Check sheet for the modelled part. Datum: model origin and axes. Units: mm. Face numbers are marked on the shaded views. Give positions to 0.01 mm unless a question says otherwise; leave off trailing zeros. Write each loop counter-clockwise with the first axis right and the second up, starting at its lowest first coordinate (ties: lowest second). Pieces come first, ordered by that corner, then holes. Notation, with made-up numbers: (-19, 58.25) -> (2, 58.25) arc R27 cw to (2, 84.25) -> close; hole circle Ø3 at (-34.75, 57.25). An arc over 180 degrees is marked (long way). Return JSON: item names as keys, results as strings.
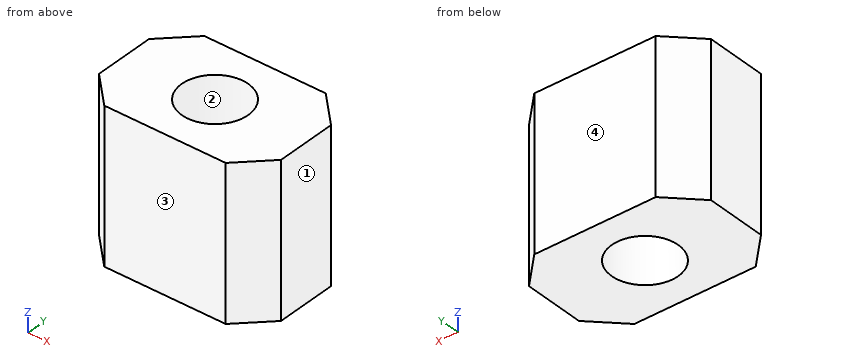
Autodesk Inventor part; units mm, degrees
ref_plane "YZ Plane" through (0, 0, 0) normal (1, 0, 0) x (0, 1, 0)
ref_plane "XZ Plane" through (0, 0, 0) normal (0, 1, 0) x (-1, 0, 0)
ref_plane "XY Plane" through (0, 0, 0) normal (0, 0, 1) x (1, 0, 0)
sketch "Sketch1" plane through (0, 0, 0) normal (0, 0, 1) x (1, 0, 0)
  line L0 (-6, 4) -> (6, 4)
  line L1 (6, 4) -> (6, -4)
  line L2 (6, -4) -> (-6, -4)
  line L3 (-6, -4) -> (-6, 4)
  line L4 (-6, 4) -> (6, -4) construction
  line L5 (6, 4) -> (-6, -4) construction
  point P0 (0, 0)
  dimension "d0" = 12
  dimension "d1" = 8
extrude "Extrusion1" add sketch "Sketch1" along normal mid plane 10
chamfer "Chamfer1" distance 2 angle 45 4 edges at (6, 4, 0) (-6, 4, 0) (-6, -4, 0) (6, -4, 0)
sketch "Sketch2" plane through (0, 0, -5) normal (0, 0, -1) x (-1, 0, 0)
  circle A0 centre (0, 0) radius 2.1875
  dimension "d7" = 4.375
extrude "Extrusion2" cut sketch "Sketch2" against normal through all
properties part number "conexion-engrane-hombro"
(1) Cross-section at B-B on x = 0. Enter the section's corners in (y, z), then the cut area to 4 significant figures.
Reply:
{"outline": "(-4, -5) -> (-2.19, -5) -> (-2.19, 5) -> (-4, 5) -> close; (2.19, -5) -> (4, -5) -> (4, 5) -> (2.19, 5) -> close", "area": "36.25 mm^2"}
(2) Cross-section at D-D on x = 4.25. Enter the section's corners in (y, z), then the cut area to 3 significant figures.
Reply:
{"outline": "(-3.75, -5) -> (3.75, -5) -> (3.75, 5) -> (-3.75, 5) -> close", "area": "75.0 mm^2"}
(3) Release check for a two-part mould opening along Y. For the marked faces 1, 2, 3 and 4 record: pulls with the +Y half, pulls with the -Y half, needs draft (parallel to the pull), parting line crosses it, or undercut.
Reply:
{"face 1": "needs draft", "face 2": "undercut", "face 3": "pulls with the -Y half", "face 4": "pulls with the +Y half"}
(4) Cross-section at A-A on y = 0. Enter the section's corners in (x, z), then the cut area to 4 significant figures.
Reply:
{"outline": "(-6, -5) -> (-2.19, -5) -> (-2.19, 5) -> (-6, 5) -> close; (2.19, -5) -> (6, -5) -> (6, 5) -> (2.19, 5) -> close", "area": "76.25 mm^2"}
(5) Thickness scan on L1, parallel to Y at x = 0, z = 1.5; L2, parallel to X at y = -3, z = 3.5; L3, parallel to X at y = 1, z = -1.75. Record the ranges inside material, lowest first.
Reply:
{"L1": "-4 to -2.19, 2.19 to 4", "L2": "-5 to 5", "L3": "-6 to -1.95, 1.95 to 6"}
(6) Cross-section at C-C on z = 0.5. Enter the section's corners in (x, y) (1 decimal), then the cut area to 3 significant figures.
Reply:
{"outline": "(-6, -2) -> (-4, -4) -> (4, -4) -> (6, -2) -> (6, 2) -> (4, 4) -> (-4, 4) -> (-6, 2) -> close; hole circle Ø4.4 at (0, 0)", "area": "73.0 mm^2"}
